Build history of the part. All positions in model axes, mm. Give positions to 0.01 mm unless a question says otherwise; leave off trailing zeros. Order: outer loops, then holes, each group sorted by start corner. A loop starts at its lowest first (then second) coordinate and runs counter-clockwise, first axis right, second up. Notation, with made-up numbers: M 14,48 L 26,48 A24 ccw 26,63 Z; hole C 1,12.25 d3. An arc over 180 degrees is marked long. One line per item, written item: value.
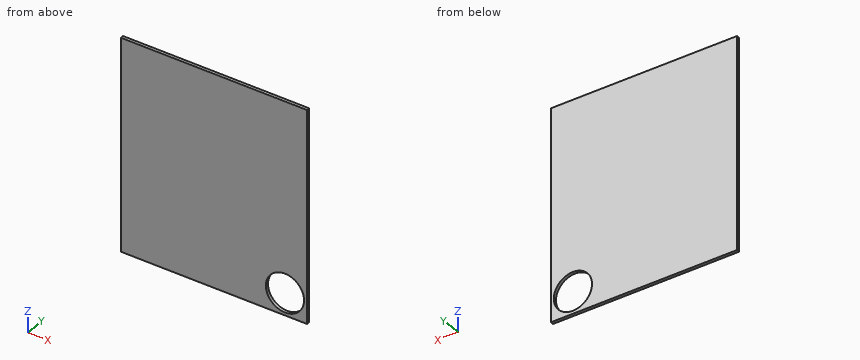
from build123d import *

# Parameters (mm, degrees)
BOSS_EXTRUDE1_DEPTH = 6.25


with BuildPart() as part:
    # Sketch1 → Boss-Extrude1 (new body)
    with BuildSketch(Plane(origin=(0, 0, 0), x_dir=(1, 0, 0), z_dir=(0, 1, 0))):
        with BuildLine():
            Line((106, 215), (106, 170))
            ThreePointArc((106, 170), (145, 209), (184, 170))
            Line((184, 170), (184, 215))
            Line((184, 215), (106, 215))
        make_face()
        with BuildLine():
            ThreePointArc((184, 170), (145, 131), (106, 170))
            Line((106, 170), (106, 215))
            Line((106, 215), (-190, 215))
            Line((-190, 215), (-190, -215))
            Line((-190, -215), (190, -215))
            Line((190, -215), (190, 215))
            Line((190, 215), (184, 215))
            Line((184, 215), (184, 170))
        make_face()
    extrude(amount=BOSS_EXTRUDE1_DEPTH)


solid = part.part
1) Saw through at A-A, the plane z = -170. Write the cut outline in (x, y).
Check values:
outline: M -190,0 L 106,0 L 106,6.25 L -190,6.25 Z; M 184,0 L 190,0 L 190,6.25 L 184,6.25 Z
2) Saw through at B-B, the plane x = 145. Write the cut outline in (y, z), then the cut area to 3 significant figures.
Check values:
outline: M 0,-215 L 6.25,-215 L 6.25,-209 L 0,-209 Z; M 0,-131 L 6.25,-131 L 6.25,215 L 0,215 Z
area: 2,200 mm^2
3) Drill centre lines: probe 1 along Z at (x, y) = (145, 3.5); probe 2 along Z at (x, y) = (143, 3.25). Where is each one in solid material? Low to high. Write a range as from..to.
Check values:
probe 1: -215..-209, -131..215
probe 2: -215..-208.95, -131.05..215
4) Pin check, flat tip, straight feed: pin 1 (10 mm diameter, centred on x = 107.5, z = 106, fed in from -Y). Stop position of the tip, or through.
Check values:
pin 1: y = 0
5) Saw through at C-C, the plane y = 1.5. Write the cut outline in (x, z), then the cut area to 3 significant figures.
Check values:
outline: M -190,-215 L 190,-215 L 190,215 L -190,215 Z; hole C 145,-170 d78
area: 159,000 mm^2
